Design review of the part shown in the three views and the two pictorial views. Dimensions are in mm from the part's minimum x, y and z. Round coordinates to 2 decimals unless told otherwise and drop trailing zeros. Loops run counter-clockwise (first coordinate to the right, second up) from the corner with the lowest first, then second, coordinate; pieces in that order, holes last. Notation, with made-up numbers: (2.5, 81) -> (42.5, 81) arc R21 ccw to (42.5, 107) -> close; hole circle Ø1 at (-26, 58.5). An arc over 180 degrees is marked (long way). Use a Markdown table: item, result. Add a question column.
1) Consider section A-A on z = 1.1. Give the boundary of the cut face in (x, y), plus the area to 3 significant figures.
2) Consider section B-B on y = 65.5. Give the boundary of the cut face in (x, z), plus the area to 3 significant figures.
3) Wall thickness on probe 1 along Y at (x, z) = (175, 2.45); probe 2 along X at (y, z) = (71, 2.15); probe 3 along X at (y, z) = (39.5, 0.2): over which ranges is each line inside the solid? List them lowest first.
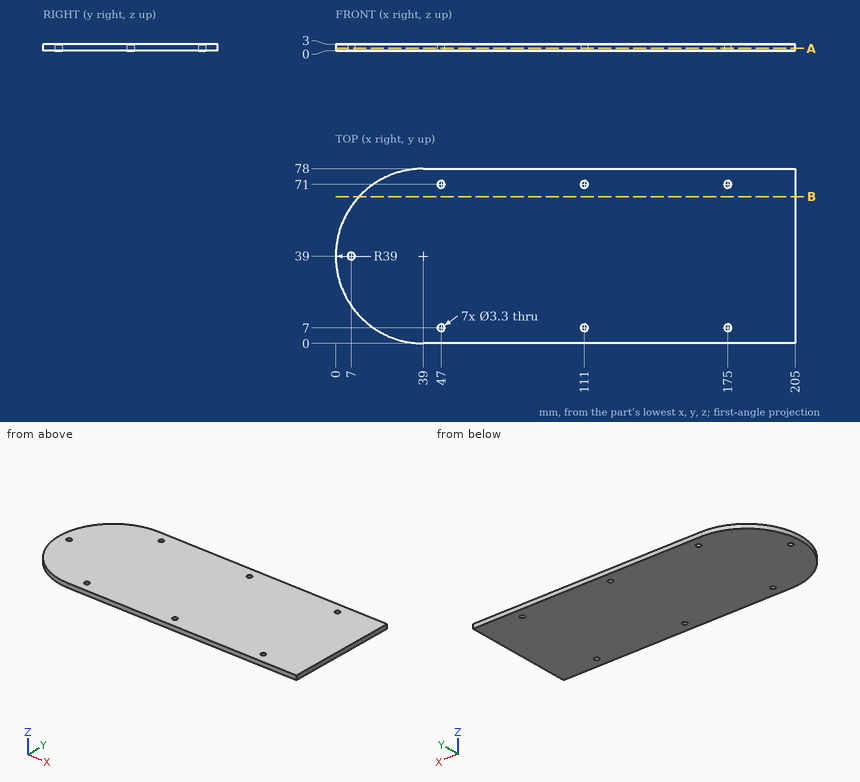
Result set:
| question | item | result |
|---|---|---|
| 1 | outline | (39, 0) -> (205, 0) -> (205, 78) -> (39, 78) arc R39 ccw to start; hole circle Ø3.3 at (7, 39); hole circle Ø3.3 at (47, 7); hole circle Ø3.3 at (47, 71); hole circle Ø3.3 at (111, 7); hole circle Ø3.3 at (111, 71); hole circle Ø3.3 at (175, 7); hole circle Ø3.3 at (175, 71) |
| 1 | area | 15,300 mm2 |
| 2 | outline | (10.39, 0) -> (205, 0) -> (205, 3) -> (10.39, 3) -> close |
| 2 | area | 584 mm2 |
| 3 | probe 1 | 0 to 5.35, 8.65 to 69.35, 72.65 to 78 |
| 3 | probe 2 | 16.71 to 45.35, 48.65 to 109.35, 112.65 to 173.35, 176.65 to 205 |
| 3 | probe 3 | 0 to 5.43, 8.57 to 205 |
